```python
from build123d import *

# Parameters (mm, degrees)
F1_DEPTH = 3
F2_ANGLE = 90
F7_W     = 20
F7_H     = 3
F8_DEPTH = 15


# Not quite as in the source:
# - ends of sketch curves that miss each other by under 0.0002 mm in the source are joined


with BuildPart() as f1:
    # F0 (on Top) → F1 (new body)
    with BuildSketch(Plane.XY):
        with BuildLine():
            ThreePointArc((2.5843454528, -32.7194872419), (1.4841670751, -33.7858704597), (0, -34.1664144431))
            Line((0, -34.1664144431), (0, -54.1664144431))
            Line((0, -54.1664144431), (30.1699284464, -54.1664144431))
            Line((30.1699284464, -54.1664144431), (30.1699284464, 31.83347))
            Line((30.1699284464, 31.83347), (0, 31.83347))
            Line((0, 31.83347), (0, 11.83347))
            ThreePointArc((0, 11.83347), (7.4846118013, 9.165784114), (11.5946270955, 2.3655094074))
            ThreePointArc((11.5946270955, 2.3655094074), (12.4147060347, -3.2443514979), (12.338869311, -8.913329936))
            ThreePointArc((12.338869311, -8.913329936), (8.8720047217, -21.3943156457), (2.5843454528, -32.7194872419))
        make_face()
    extrude(amount=F1_DEPTH)


with BuildPart() as f1_1:
    # F2: moved
    add(f1.part.rotate(Axis((0, -44.1664144431, 3), (0, -1, 0)), F2_ANGLE))

    # F7 (on 3pt) → F8 (join, symmetric)
    with BuildSketch(Plane.YZ.offset(1.5)):
        with Locations((-44.1664144431, 4.5)):
            Rectangle(F7_W, F7_H)
        with Locations((21.83347, 4.5)):
            Rectangle(F7_W, F7_H)
    extrude(amount=F8_DEPTH, both=True)


solid = f1_1.part
```
Read the model definition and answer for the solid it produces. Units are mm, in the model's axes. A direction names the side the tool comes from. Coordinates: 2 decimals unless noted, no trailing zeros. Write each loop counter-clockwise with the first axis right and the second up, starting at its lowest first coordinate (ties: lowest second). Pieces come first, ordered by that corner, then holes. Notation, with made-up numbers: (85, 71) -> (102, 71) arc R18 ccw to (102, 88) -> close; hole circle Ø2 at (-17.5, 42). An arc over 180 degrees is marked (long way). Answer as a JSON object with one key per item and string values.
Q1. A tool of negligible diameter and unlimited length cuts with its end or side. For faces 4 (the cylindrical face through (1.521, 9.237, 10.396)), 5 (the flat face through (10, 11.833, 4)), 6 (the flat face through (10, 22, 6)), from which of +Z, -Z, +X, -X, +Y, -Y can it reach the whole face along a straight path? Write none if from no direction.
The answers:
{"face 4": "-Z, +X, -X", "face 5": "+Z, -Z, +X", "face 6": "+Z, +X, +Y, -Y"}
Q2. Consider line 1 (X direction, y = -49.5, z = 11.5); line 2 (Y direction, x = 5.5, z = 5.5); line 3 (Z direction, x = 13.5, y = -45.5). Determine where each line is inside the solid, lowest interval first. Write a range as [from, to].
The answers:
{"line 1": "x = [0, 3]", "line 2": "y = [-54.17, -34.17], [11.83, 31.83]", "line 3": "z = [3, 6]"}
Q3. The part is cut by section D-D on y = -15. Give the vertices of the cut face in (x, z), then the cut area to 3 significant figures.
The answers:
{"outline": "(0, 14.04) -> (3, 14.04) -> (3, 33.17) -> (0, 33.17) -> close", "area": "57.4 mm2"}
Q4. The part is cut by section A-A on x = -9.25. Give the vertices of the cut face in (y, z), then the cut area to 3 significant figures.
The answers:
{"outline": "(-54.17, 3) -> (-34.17, 3) -> (-34.17, 6) -> (-54.17, 6) -> close; (11.83, 3) -> (31.83, 3) -> (31.83, 6) -> (11.83, 6) -> close", "area": "120 mm2"}
Q5. Determine the mould class of faces 1 (the flat face through (16.5, 22, 5)), 2 (the flat face through (-2, -34.166, 4)), 3 (the flat face through (-13.5, -44, 5)) for opening direction X: pulls with the +X half, pulls with the -X half, needs draft (parallel to the pull), parting line crosses it, or undercut.
The answers:
{"face 1": "pulls with the +X half", "face 2": "needs draft", "face 3": "pulls with the -X half"}
Q6. The part is cut by section B-B on x = 1.75. Give the vertices of the cut face in (y, z), then the cut area to 3 significant figures.
The answers:
{"outline": "(-54.17, 3) -> (-34.17, 3) -> (-34.17, 3.05) arc R2.99 cw to (-32.72, 5.58) arc R55.04 cw to (-8.91, 15.34) arc R35.8 cw to (2.37, 14.59) arc R11.83 cw to (11.83, 3) -> (31.83, 3) -> (31.83, 33.17) -> (-54.17, 33.17) -> close", "area": "2,170 mm2"}
Q7. Flat-ended cylindrical pins translate along their axes: pin 1 Ø6 at (x, y) = (6.5, -17) entering from +Z; pin 2 Ø7 at (x, y) = (7, 22) entering from +Z; pin 3 Ø1 at (y, z) = (-29.5, 28) entering from -X; pin 4 Ø4 at (y, z) = (-12, 26) entering from +X. Find the tip coordinate at first contact, or state that the pin passes through.
The answers:
{"pin 1": "passes through", "pin 2": "stops at z = 6", "pin 3": "stops at x = 0", "pin 4": "stops at x = 3"}
Q8. The part is cut by section C-C on z = 23. Give the vertices of the cut face in (x, y), then the cut area to 3 significant figures.
The answers:
{"outline": "(0, -54.17) -> (3, -54.17) -> (3, 31.83) -> (0, 31.83) -> close", "area": "258 mm2"}
